Model file for the job. Use its own axes, mm. A direction names the side the tool comes from. Round coordinates to 2 decimals unless told otherwise and drop trailing zeros. Loops run counter-clockwise (first coordinate to the right, second up) from the corner with the lowest first, then second, coordinate; pieces in that order, holes last. Notation, with made-up numbers: M -11,13.5 L 11,13.5 A13 cw 11,24.5 Z; hole C 33.25,77 d6. An arc over 180 degrees is marked long. Answer in a Markdown table with one row per item.
from build123d import *

# Parameters (mm, degrees)
SKETCH_1_W      = 62
SKETCH_1_H      = 81
SKETCH_1_W_2    = 54
SKETCH_1_H_2    = 73
EXTRUDE_1_DEPTH = 2
EXTRUDE_2_DEPTH = 4
EXTRUDE_3_DEPTH = 4
EXTRUDE_4_DEPTH = 4
EXTRUDE_5_DEPTH = 4
EXTRUDE_6_DEPTH = 4
EXTRUDE_7_DEPTH = 4
EXTRUDE_8_DEPTH = 4
EXTRUDE_9_DEPTH = 4


with BuildPart() as part:
    # Эскиз1 → Бобышка-Вытянуть1 (new body)
    with BuildSketch(Plane(origin=(0, 0, 0), x_dir=(1, 0, 0), z_dir=(0, 1, 0))):
        Rectangle(SKETCH_1_W, SKETCH_1_H)
        Rectangle(SKETCH_1_W_2, SKETCH_1_H_2, mode=Mode.SUBTRACT)
    extrude(amount=EXTRUDE_1_DEPTH)

    # Эскиз6 → Бобышка-Вытянуть2 (add)
    with BuildSketch(Plane.XY.offset(40.5)):
        Polygon((26, 2), (31, 2), (31, 8), (26, 8), (26, 6), (29, 6), (29, 4.9), (26, 4.9), align=None)
        Polygon((21, 2), (26, 2), (26, 4.9), align=None)
    extrude(amount=-EXTRUDE_2_DEPTH)

    # Эскиз8 → Бобышка-Вытянуть3 (add)
    with BuildSketch(Plane.XY.offset(40.5)):
        Polygon((-31, 8), (-31, 2), (-26, 2), (-26, 4.9), (-29, 4.9), (-29, 6), (-26, 6), (-26, 8), align=None)
        Polygon((-26, 4.9), (-26, 2), (-21, 2), align=None)
    extrude(amount=-EXTRUDE_3_DEPTH)

    # Эскиз10 → Бобышка-Вытянуть4 (add)
    with BuildSketch(Plane(origin=(0, 0, -40.5), x_dir=(-1, 0, 0), z_dir=(0, 0, -1))):
        Polygon((-31, 8), (-31, 2), (-24, 2), (-24, 4.9), (-29, 5), (-29, 6), (-26, 6), (-26, 8), align=None)
        Polygon((-24, 4.9), (-24, 2), (-21, 2), align=None)
    extrude(amount=-EXTRUDE_4_DEPTH)

    # Эскиз11 → Бобышка-Вытянуть5 (add)
    with BuildSketch(Plane(origin=(0, 0, -40.5), x_dir=(-1, 0, 0), z_dir=(0, 0, -1))):
        Polygon((24, 2), (31, 2), (31, 8), (26, 8), (26, 6), (29, 6), (29, 4.9), (24, 4.9), align=None)
        Polygon((21, 2), (24, 2), (24, 4.9), align=None)
    extrude(amount=-EXTRUDE_5_DEPTH)

    # Эскиз12 → Бобышка-Вытянуть6 (add)
    with BuildSketch(Plane.ZY.offset(31)):
        Polygon((-36.5, 2), (-31.5, 2), (-36.5, 4.866692533), align=None)
    extrude(amount=-EXTRUDE_6_DEPTH)

    # Эскиз13 → Бобышка-Вытянуть7 (add)
    with BuildSketch(Plane.ZY.offset(31)):
        Polygon((36.5, 2), (36.5, 5), (31.5, 2), align=None)
    extrude(amount=-EXTRUDE_7_DEPTH)

    # Эскиз17 → Бобышка-Вытянуть8 (add)
    with BuildSketch(Plane(origin=(31, 0, 0), x_dir=(0, 0, -1), z_dir=(1, 0, 0))):
        Polygon((-31.5, 2), (-36.5, 4.867780804), (-36.5, 2), align=None)
    extrude(amount=-EXTRUDE_8_DEPTH)

    # Эскиз21 → Бобышка-Вытянуть9 (add)
    with BuildSketch(Plane(origin=(31, 0, 0), x_dir=(0, 0, -1), z_dir=(1, 0, 0))):
        Polygon((36.5, 2), (36.5, 4.866692533), (31.5, 2), align=None)
    extrude(amount=-EXTRUDE_9_DEPTH)


solid = part.part
1. Pin check, flat tip, straight feed: pin 1 (2 mm diameter, centred on x = -29, z = 1.5, fed in from +Y). Stop position of the tip, or through.
Verdict:
| item | result |
|---|---|
| pin 1 | stops at y = 2 |
2. Mould opens along X. For faces 6 (the flat face through (-29, 7, 36.5)), 7 (the flat face through (-31, 1, 0)), 8 (the flat face through (28, 6, -39)), 9 (the flat face through (0, 2, -39)) say: +X half, -X half, draft (parallel to the pull), parting line (faces both ways), or undercut.
Verdict:
| item | result |
|---|---|
| face 6 | draft |
| face 7 | -X half |
| face 8 | undercut |
| face 9 | undercut |
3. Saw through at C-C (y = 7). Write the cut outline in (x, z).
Verdict:
| item | result |
|---|---|
| outline | M -31,-40.5 L -26,-40.5 L -26,-36.5 L -31,-36.5 Z; M -31,36.5 L -26,36.5 L -26,40.5 L -31,40.5 Z; M 26,-40.5 L 31,-40.5 L 31,-36.5 L 26,-36.5 Z; M 26,36.5 L 31,36.5 L 31,40.5 L 26,40.5 Z |
4. Saw through at A-A (x = 15). Write the cut outline in (y, z), and give its area (3 significant figures).
Verdict:
| item | result |
|---|---|
| outline | M 0,-40.5 L 2,-40.5 L 2,-36.5 L 0,-36.5 Z; M 0,36.5 L 2,36.5 L 2,40.5 L 0,40.5 Z |
| area | 16.0 mm² |
5. Tool access for faces 1 (the flat face through (-26, 7, 39)), 2 (the flat face through (29.028, 3.414, 33.965)), 3 (the flat face through (-28, 6, 39)), 4 (the flat face through (-29, 2, 0)), 5 (the flat face through (-27, 1, -1)): list every direction of +Z, -Z, +X, -X, +Y, -Y with a clear straight run to the whole face (end or side of a thin tool).
Verdict:
| item | result |
|---|---|
| face 1 | +Z, -Z, +Y |
| face 2 | +X, +Y |
| face 3 | +Z, -Z |
| face 4 | +X, -X, +Y |
| face 5 | +Y, -Y |
6. Wall check: probe 1 along Z at (x, y) = (-5, 0.5); probe 2 along X at (y, z) = (0.5, 19). Give the ranges that are in metal, low to high.
Verdict:
| item | result |
|---|---|
| probe 1 | z = -40.5 to -36.5, 36.5 to 40.5 |
| probe 2 | x = -31 to -27, 27 to 31 |
7. Saw through at B-B (z = 1). Write the cut outline in (x, y), and give its area (3 significant figures).
Verdict:
| item | result |
|---|---|
| outline | M -31,0 L -27,0 L -27,2 L -31,2 Z; M 27,0 L 31,0 L 31,2 L 27,2 Z |
| area | 16.0 mm² |
